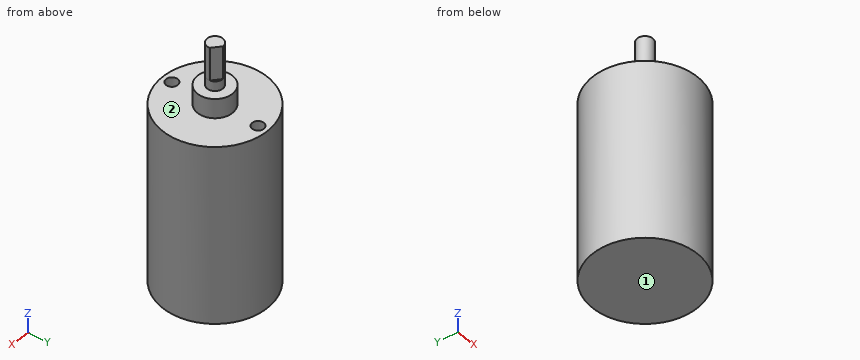
from build123d import *

# Parameters (mm, degrees)
SCHIZZO1_R                   = 13.5
ESTRUSIONE_ESTRUSIONE1_DEPTH = 46
SCHIZZO2_R                   = 4.5
ESTRUSIONE_ESTRUSIONE2_DEPTH = 5
SCHIZZO4_R                   = 2
ESTRUSIONE_ESTRUSIONE3_DEPTH = 2.5
ESTRUSIONE_ESTRUSIONE4_DEPTH = 8.5
SCHIZZO6_R                   = 1.5
TAGLIO_ESTRUSIONE1_DEPTH     = 10


with BuildPart() as part:
    # Schizzo1 → Estrusione-Estrusione1 (new body)
    with BuildSketch(Plane.XY):
        Circle(SCHIZZO1_R)
    extrude(amount=ESTRUSIONE_ESTRUSIONE1_DEPTH)

    # Schizzo2 → Estrusione-Estrusione2 (add)
    with BuildSketch(Plane.XY.offset(46)):
        Circle(SCHIZZO2_R)
    extrude(amount=ESTRUSIONE_ESTRUSIONE2_DEPTH)

    # Schizzo4 → Estrusione-Estrusione3 (add)
    with BuildSketch(Plane.XY.offset(51)):
        Circle(SCHIZZO4_R)
    extrude(amount=ESTRUSIONE_ESTRUSIONE3_DEPTH)

    # Schizzo5 → Estrusione-Estrusione4 (add)
    with BuildSketch(Plane.XY.offset(53.5)):
        with BuildLine():
            Line((1.984313483, 0.25), (0, 2))
            ThreePointArc((0, 2), (-1.414213562, -1.414213562), (2, 0))
            ThreePointArc((2, 0), (1.996074518, 0.125245825), (1.984313483, 0.25))
        make_face()
    extrude(amount=ESTRUSIONE_ESTRUSIONE4_DEPTH)

    # Schizzo6 → Taglio-Estrusione1 (cut)
    with BuildSketch(Plane.XY.offset(46)):
        with Locations((0, 11)):
            Circle(SCHIZZO6_R)
        with Locations((0, -11)):
            Circle(SCHIZZO6_R)
    extrude(amount=-TAGLIO_ESTRUSIONE1_DEPTH, mode=Mode.SUBTRACT)


solid = part.part
Geometry: final body of the model. Coordinates: model frame, mm. Face numbers are marked on the shaded views. A direction names the side the tool comes from. Round coordinates to 2 decimals unless told otherwise and drop trailing zeros. Loops run counter-clockwise (first coordinate to the right, second up) from the corner with the lowest first, then second, coordinate; pieces in that order, holes last. Notation, with made-up numbers: (36.5, 36.25) -> (53.5, 36.25) arc R27 cw to (53.5, 70.25) -> close; hole circle Ø5 at (22.5, 11). An arc over 180 degrees is marked (long way). One line per question, with ' | ' between items. Start each with the question number.
1. Section D-D on x = 8.75. Output: boundary loops of the cut face in (y, z).
2. Set-up query: the marked faces 1 and 2. Return all of +Z, -Z, +X, -X, +Y, -Y with unobstructed straight access to the full face (end or side cutting, diameter ignored); none if empty.
3. Line query: line 1 along Y through (x, z) = (0, 41.5); line 2 along Z through (x, y) = (6.5, -10.25); line 3 along Z through (x, y) = (2.25, 3.75). Output: solid intervals per line, ascending. Write a range as [from, to].
4. Contact query for flat-ended pins moving along their axis: pin 1 (2.5 mm diameter, centred on x = 0.5, y = 11.5, fed in from +Z); pin 2 (8 mm diameter, centred on x = -1, y = -6.5, fed in from +Z); pin 3 (2 mm diameter, centred on x = -1.5, z = 25.5, fed in from -Y). Output: stop coordinate, or through.
5. Section B-B on y = 11. Output: boundary loops of the cut face in (x, z), and give its area (3 significant figures).
6. Section A-A on z = 39. Output: boundary loops of the cut face in (x, y).
7. Section C-C on z = 48.5. Output: boundary loops of the cut face in (x, y).
Returned:
1) outline: (-10.28, 0) -> (10.28, 0) -> (10.28, 46) -> (-10.28, 46) -> close
2) face 1: -Z, +X, -X, +Y, -Y | face 2: +Z
3) line 1: y = [-13.5, -12.5], [-9.5, 9.5], [12.5, 13.5] | line 2: z = [0, 46] | line 3: z = [0, 51]
4) pin 1: stops at z = 46 | pin 2: stops at z = 51 | pin 3: stops at y = -13.49
5) outline: (-7.83, 0) -> (7.83, 0) -> (7.83, 46) -> (1.5, 46) -> (1.5, 36) -> (-1.5, 36) -> (-1.5, 46) -> (-7.83, 46) -> close | area: 690 mm2
6) outline: circle Ø27 at (0, 0); hole circle Ø3 at (0, -11); hole circle Ø3 at (0, 11)
7) outline: circle Ø9 at (0, 0)
